Answer from the drawing. Dimensions are ordinates in mm from the lowest x, y and z of the part. Give positions to 0.01 mm unless a question says otherwise; leave off trailing zeros. Write each loop counter-clockwise with the first axis right and the second up, starting at its lowest first coordinate (ties: lowest second). Pieces come first, ordered by that corner, then holes. Notation, with made-up numbers: M 15.25,77 L 41.25,77 A18 cw 41.25,98 Z; hole C -21.75,25.5 d5. An arc over 180 degrees is marked long. Write each question's results on one line, items separated by ' | '. Start each with the question number.
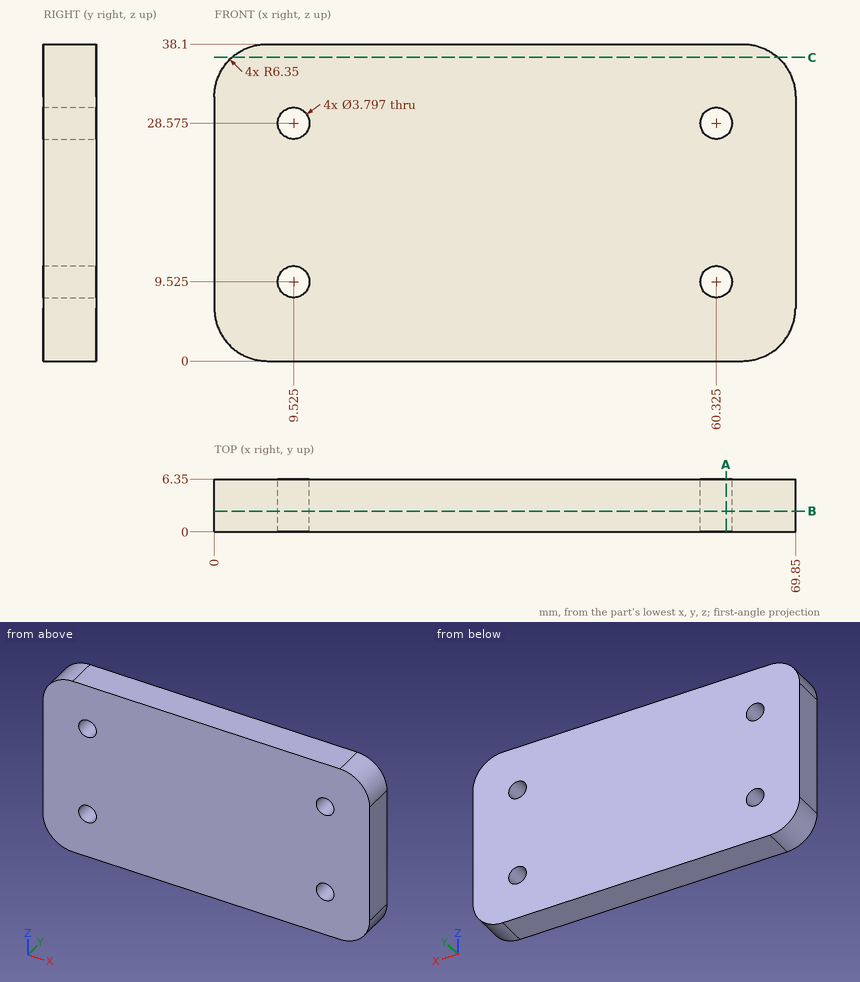
Item 1: Section C-C, the plane z = 36.5 is taken. Determine the outline of the cut face in (x, y).
Item 2: Section B-B, the plane y = 2.5 is taken. Give the number of separate pieces and of enclosed holes in the cut face, then the cut area to 3 significant figures.
Item 3: Section A-A, the plane x = 61.5 is taken. Determine the outline of the cut face in (y, z), then the cut area to 3 significant figures.
Item 4: Straight lines are drawn through the part: line 1 (Z direction, x = 59, y = 4) (1 decimal); line 2 (X direction, y = 2.75, z = 9); line 3 (X direction, y = 5.5, z = 10). For each, find the intervals that lie inside material, in ascending order.
Worked out:
1) outline: M 2.14,0 L 67.71,0 L 67.71,6.35 L 2.14,6.35 Z
2) separate pieces: 1 | enclosed holes: 4 | area: 2,580 mm²
3) outline: M 0,0 L 6.35,0 L 6.35,8.03 L 0,8.03 Z; M 0,11.02 L 6.35,11.02 L 6.35,27.08 L 0,27.08 Z; M 0,30.07 L 6.35,30.07 L 6.35,38.1 L 0,38.1 Z | area: 204 mm²
4) line 1: z = 0 to 8.2, 10.9 to 27.2, 29.9 to 38.1 | line 2: x = 0 to 7.7, 11.35 to 58.5, 62.15 to 69.85 | line 3: x = 0 to 7.69, 11.36 to 58.49, 62.16 to 69.85
